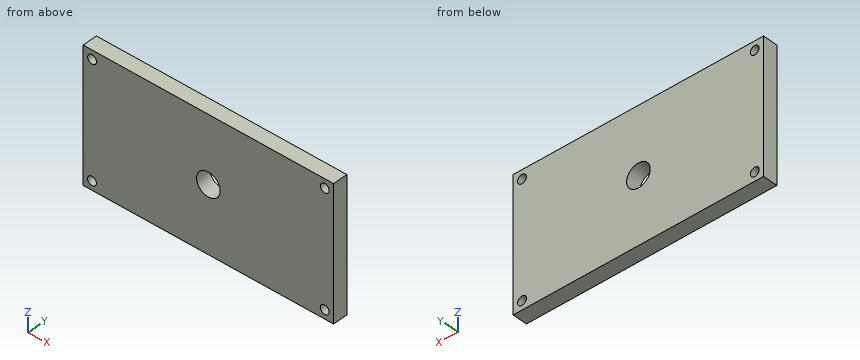
```python
from build123d import *

# Parameters (mm, degrees)
SKETCH1_W           = 85
SKETCH1_H           = 45
BOSS_EXTRUDE1_DEPTH = 5
SKETCH2_R           = 1.5
CUT_EXTRUDE1_DEPTH  = 5
SKETCH3_R           = 4
CUT_EXTRUDE2_DEPTH  = 10


with BuildPart() as part:
    # Sketch1 → Boss-Extrude1 (new body)
    with BuildSketch(Plane(origin=(0, 0, 0), x_dir=(1, 0, 0), z_dir=(0, 1, 0))):
        with Locations((42.5, 22.5)):
            Rectangle(SKETCH1_W, SKETCH1_H)
    extrude(amount=BOSS_EXTRUDE1_DEPTH)

    # Sketch2 → Cut-Extrude1 (cut)
    with BuildSketch(Plane(origin=(0, 5, 0), x_dir=(1, 0, 0), z_dir=(0, 1, 0))):
        with Locations(Location((3, 42, 0), (0, 0, 270))):
            Circle(SKETCH2_R)
        with Locations(Location((3, 3, 0), (0, 0, 270))):
            Circle(SKETCH2_R)
        with Locations(Location((82, 3, 0), (0, 0, 270))):
            Circle(SKETCH2_R)
        with Locations(Location((82, 42, 0), (0, 0, 270))):
            Circle(SKETCH2_R)
    extrude(amount=-CUT_EXTRUDE1_DEPTH, mode=Mode.SUBTRACT)

    # Sketch3 → Cut-Extrude2 (cut)
    with BuildSketch(Plane(origin=(0, 5, 0), x_dir=(1, 0, 0), z_dir=(0, 1, 0))):
        with Locations(Location((42.5, 22.5, 0), (0, 0, 270))):
            Circle(SKETCH3_R)
    extrude(amount=-CUT_EXTRUDE2_DEPTH, mode=Mode.SUBTRACT)


solid = part.part
```
Source: CAD feature listing. Evaluate the final solid. Frame: model axes, mm. Round coordinates to 2 decimals unless told otherwise and drop trailing zeros. Write each loop counter-clockwise with the first axis right and the second up, starting at its lowest first coordinate (ties: lowest second). Pieces come first, ordered by that corner, then holes. Notation, with made-up numbers: M 33,28.5 L 72,28.5 A5 cw 72,37.5 Z; hole C 85,-27.5 d7. An arc over 180 degrees is marked long. Answer as a JSON object with one key per item and string values. Group by question number.
(1) Ray query, line 1 (X direction, y = 1.2, z = -3); line 2 (X direction, y = 2.3, z = -22.5); line 3 (Z direction, x = 82, y = 2.4). Return the intervals inside material, ascending. Write a range as [from, to].
(2) Section query D-D on x = 45.5. Output: boundary loops of the cut face in (y, z).
(3) Section query B-B on x = 82. Output: boundary loops of the cut face in (y, z).
(4) Section query C-C on y = 1. Output: boundary loops of the cut face in (x, z), then the cut area to 3 significant figures.
(5) Section query A-A on z = -42. Output: boundary loops of the cut face in (x, y).
Computed values:
{
 "1": {"line 1": "[0, 1.5], [4.5, 80.5], [83.5, 85]", "line 2": "[0, 38.5], [46.5, 85]", "line 3": "[-45, -43.5], [-40.5, -4.5], [-1.5, 0]"},
 "2": {"outline": "M 0,-45 L 5,-45 L 5,-25.15 L 0,-25.15 Z; M 0,-19.85 L 5,-19.85 L 5,0 L 0,0 Z"},
 "3": {"outline": "M 0,-45 L 5,-45 L 5,-43.5 L 0,-43.5 Z; M 0,-40.5 L 5,-40.5 L 5,-4.5 L 0,-4.5 Z; M 0,-1.5 L 5,-1.5 L 5,0 L 0,0 Z"},
 "4": {"outline": "M 0,-45 L 85,-45 L 85,0 L 0,0 Z; hole C 3,-42 d3; hole C 3,-3 d3; hole C 42.5,-22.5 d8; hole C 82,-42 d3; hole C 82,-3 d3", "area": "3,750 mm^2"},
 "5": {"outline": "M 0,0 L 1.5,0 L 1.5,5 L 0,5 Z; M 4.5,0 L 80.5,0 L 80.5,5 L 4.5,5 Z; M 83.5,0 L 85,0 L 85,5 L 83.5,5 Z"}
}
